from build123d import *

# Parameters (mm, degrees)
ESBO_O1_W                = 55.5
ESBO_O1_H                = 55.5
RESSALTO_EXTRUS_O1_DEPTH = 2.5
FILETE1_R                = 3
FILETE2_R                = 3
FILETE3_R                = 3
FILETE4_R                = 3
ESBO_O3_W                = 4.3
ESBO_O3_H                = 7
ESBO_O3_W_2              = 7
ESBO_O3_H_2              = 4.3
CORTE_EXTRUS_O1_DEPTH    = 40.323974875


with BuildPart() as part:
    # Esboço1 → Ressalto-extrusão1 (new body)
    with BuildSketch(Plane(origin=(0, 0, 0), x_dir=(1, 0, 0), z_dir=(0, 1, 0))):
        Rectangle(ESBO_O1_W, ESBO_O1_H)
    extrude(amount=RESSALTO_EXTRUS_O1_DEPTH)

    # Filete1
    filete1_edges = [part.edges().sort_by_distance(p)[0] for p in [
        (27.75, 1.25, -27.75),
    ]]
    fillet(filete1_edges, radius=FILETE1_R)

    # Filete2
    filete2_edges = [part.edges().sort_by_distance(p)[0] for p in [
        (-27.75, 1.25, -27.75),
    ]]
    fillet(filete2_edges, radius=FILETE2_R)

    # Filete3
    filete3_edges = [part.edges().sort_by_distance(p)[0] for p in [
        (-27.75, 1.25, 27.75),
    ]]
    fillet(filete3_edges, radius=FILETE3_R)

    # Filete4
    filete4_edges = [part.edges().sort_by_distance(p)[0] for p in [
        (27.75, 1.25, 27.75),
    ]]
    fillet(filete4_edges, radius=FILETE4_R)

    # Esboço3 → Corte-extrusão1 (cut, through all)
    with BuildSketch(Plane(origin=(0, 2.5, 0), x_dir=(1, 0, 0), z_dir=(0, 1, 0))):
        with Locations((0, 5.65)):
            Rectangle(ESBO_O3_W, ESBO_O3_H)
        with Locations((-5.65, 0)):
            Rectangle(ESBO_O3_W_2, ESBO_O3_H_2)
        with Locations((0, -5.65)):
            Rectangle(ESBO_O3_W, ESBO_O3_H)
        Rectangle(ESBO_O3_W, ESBO_O3_H_2)
        with Locations((5.65, 0)):
            Rectangle(ESBO_O3_W_2, ESBO_O3_H_2)
    extrude(amount=-CORTE_EXTRUS_O1_DEPTH, mode=Mode.SUBTRACT)


solid = part.part
The model under review builds one solid part; all positions refer to its coordinate system, in mm. A direction names the side the tool comes from. Coordinates: 2 decimals unless noted, no trailing zeros. Order: outer loops, then holes, each group sorted by start corner. A loop starts at its lowest first (then second) coordinate and runs counter-clockwise, first axis right, second up. Notation, with made-up numbers: (60, 26.5) -> (83, 26.5) arc R16 cw to (83, 35.5) -> close; hole circle Ø9 at (44, 76). An arc over 180 degrees is marked (long way). Answer in a Markdown table with one row per item.
(1) The part is to be moulded in two halves that separate along X. For faces 1 (the flat face through (2.15, 1, 6)), 2 (the cylindrical face through (-26.89, 1.27, 26.85)), 3 (the flat face through (0, 1, 27.75)), say which applies: +X half, -X half, draft (parallel to the pull), parting line (faces both ways), or undercut.
Answers:
| item | result |
|---|---|
| face 1 | undercut |
| face 2 | -X half |
| face 3 | draft |
(2) Machinability: for faces 4 (the flat face through (0, 1, 9.15)), 5 (the flat face through (6, 0, -7)), which of the approach directions +Z, -Z, +X, -X, +Y, -Y give a long, thin tool a straight path to every point of the face, cutting with its end or side? Answer none if there is none.
Answers:
| item | result |
|---|---|
| face 4 | +Y, -Y |
| face 5 | +Z, -Z, +X, -X, -Y |
(3) Consider section B-B (x = 4). Write out the cut boundary in (y, z).
Answers:
| item | result |
|---|---|
| outline | (0, -27.75) -> (2.5, -27.75) -> (2.5, -2.15) -> (0, -2.15) -> close; (0, 2.15) -> (2.5, 2.15) -> (2.5, 27.75) -> (0, 27.75) -> close |
(4) Consider section A-A (z = -8). Write out the cut boundary in (x, y), plus the area to 3 significant figures.
Answers:
| item | result |
|---|---|
| outline | (-27.75, 0) -> (-2.15, 0) -> (-2.15, 2.5) -> (-27.75, 2.5) -> close; (2.15, 0) -> (27.75, 0) -> (27.75, 2.5) -> (2.15, 2.5) -> close |
| area | 128 mm² |
(5) Consider section C-C (y = 1.65). Write out the cut boundary in (x, z), plus the area to 3 significant figures.
Answers:
| item | result |
|---|---|
| outline | (-27.75, -24.75) arc R3 ccw to (-24.75, -27.75) -> (24.75, -27.75) arc R3 ccw to (27.75, -24.75) -> (27.75, 24.75) arc R3 ccw to (24.75, 27.75) -> (-24.75, 27.75) arc R3 ccw to (-27.75, 24.75) -> close; hole (-9.15, -2.15) -> (-2.15, -2.15) -> (-2.15, -9.15) -> (2.15, -9.15) -> (2.15, -2.15) -> (9.15, -2.15) -> (9.15, 2.15) -> (2.15, 2.15) -> (2.15, 9.15) -> (-2.15, 9.15) -> (-2.15, 2.15) -> (-9.15, 2.15) -> close |
| area | 2,930 mm² |
(6) Wall thickness on line 1 along Z through (x, y) = (-6.5, 1.35); line 2 along X through (y, z) = (1.4, 0.5): over which ranges is each line inside the solid? List them lowest first.
Answers:
| item | result |
|---|---|
| line 1 | -27.75 to -2.15, 2.15 to 27.75 |
| line 2 | -27.75 to -9.15, 9.15 to 27.75 |
